Print and shaded views of the part. All mm, measured from the part's lowest x, y and z. Coordinates: 2 decimals unless noted, no trailing zeros. Write each loop counter-clockwise with the first axis right and the second up, starting at its lowest first coordinate (ties: lowest second). Pieces come first, ordered by that corner, then holes. Notation, with made-up numbers: (-25.75, 35.5) -> (4.25, 35.5) arc R14 ccw to (4.25, 49.5) -> close; hole circle Ø8 at (81, 47). An arc over 180 degrees is marked (long way). Write item = value, one per line.
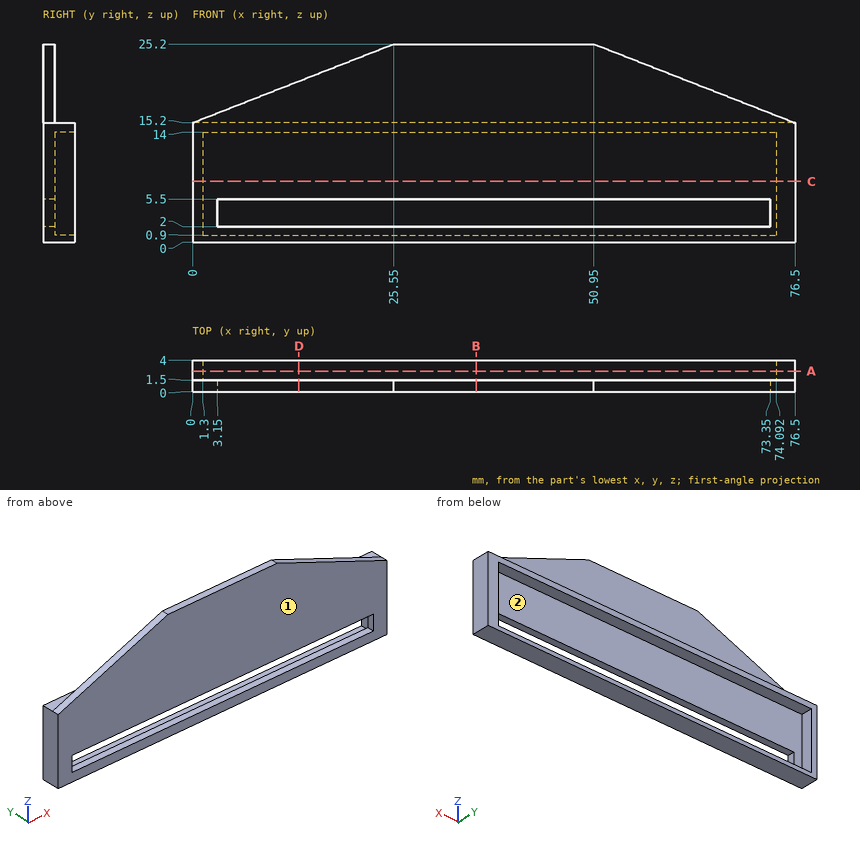
Q1. Saw through at B-B on x = 36. Give the cut face in (y, z), and give its area (3 significant figures).
Model answer:
outline = (0, 0) -> (4, 0) -> (4, 0.9) -> (1.5, 0.9) -> (1.5, 2) -> (0, 2) -> close; (0, 5.5) -> (1.5, 5.5) -> (1.5, 14) -> (4, 14) -> (4, 15.2) -> (1.5, 15.2) -> (1.5, 25.2) -> (0, 25.2) -> close
area = 37.8 mm²
Q2. Saw through at D-D on x = 13.5. Give the cut face in (y, z), and give its area (3 significant figures).
Model answer:
outline = (0, 0) -> (4, 0) -> (4, 0.9) -> (1.5, 0.9) -> (1.5, 2) -> (0, 2) -> close; (0, 5.5) -> (1.5, 5.5) -> (1.5, 14) -> (4, 14) -> (4, 15.2) -> (1.5, 15.2) -> (1.5, 20.48) -> (0, 20.48) -> close
area = 30.7 mm²
Q3. Probe line 1 (Z direction, x = 43, y = 2.1); line 2 (X direction, y = 2.3, z = 7.25); line 3 (Y direction, x = 19, z = 12.5). List the from-to ranges inside material, lowest first. Write a range as from..to.
Model answer:
line_1 = 0..0.9, 14..15.2
line_2 = 0..1.3, 74.09..76.5
line_3 = 0..1.5
Q4. Saw through at A-A on y = 2.65. Give the cut face in (x, z).
Model answer:
outline = (0, 0) -> (76.5, 0) -> (76.5, 15.2) -> (0, 15.2) -> close; hole (1.3, 0.9) -> (74.09, 0.9) -> (74.09, 14) -> (1.3, 14) -> close
Q5. Pin check, flat tips, straight feed: pin 1 (1.5 mm diameter, centred on x = 30, z = 19.5, fed in from +Y); pin 2 (1.2 mm diameter, centred on x = 23, y = 3, fed in from +Z). Stop position of each tip, or through.
Model answer:
pin_1 = 1.5
pin_2 = 15.2
Q6. Mould opens along Z. For the marked faces 1 and 2 say: released by +Z, released by -Z, zero draft, split by the parting line, or undercut.
Model answer:
face_1 = zero draft
face_2 = undercut
Q7. Saw through at C-C on z = 7.75. Give the cut face in (x, y), and give its area (3 significant figures).
Model answer:
outline = (0, 0) -> (76.5, 0) -> (76.5, 4) -> (74.09, 4) -> (74.09, 1.5) -> (1.3, 1.5) -> (1.3, 4) -> (0, 4) -> close
area = 124 mm²
